Check sheet for the modelled part. Datum: model origin and axes. Units: mm. A direction names the side the tool comes from. Round coordinates to 2 decimals unless told otherwise and drop trailing zeros. Order: outer loops, then holes, each group sorted by start corner. A loop starts at its lowest first (then second) coordinate and runs counter-clockwise, first axis right, second up.
(1) Sectioned sample at B-B, the plane z = 14.5. Enter the section's corners in (x, y).
(2) Sectioned sample at C-C, the plane x = -3. Count the separate pieces of the cut face and the enclosed holes in it, and give its area (3 significant figures).
(3) Sectioned sample at A-A, the plane x = 13. Enter the section's corners in (y, z).
(4) Thickness scan on probe 1 along Z at (x, y) = (-3, 0.5) (3 decimals); probe 2 along Z at (x, y) = (-3, 1.8) (3 decimals); probe 3 along X at (y, z) = (0.45, 16.5). Record the ranges inside material, lowest first.
(5) Depth check by flat-ended pin: pin 1 (1.8 mm diameter, centred on x = -17, z = -21.285, fed in from +Y); pin 2 (3 mm diameter, centred on x = -16.77, z = -28.78, fed in from +Y). Enter the tip coordinate at first touch or a pass-through.
(6) Tool access check on faces 4 (the flat face through (-4, 1.35, 28)), 5 (the flat face through (12, 2, 26)), 6 (the flat face through (0, 0, 10)). Record the directions out of +Z, -Z, +X, -X, +Y, -Y that give a thin tool (end or side, any length) a straight path to the whole face; none if there is none.
(7) Mould release check, pull along X, two halves, no side actions. Record for faces 1 (the cylindrical face through (-16.462, 0.684, -22.128)), 2 (the flat face through (-32, 1, -1)), 3 (the flat face through (32, 1, 1)): released by +X, released by -X, zero draft, split by the parting line, or undercut.
```python
from build123d import *

# Parameters (mm, degrees)
BOSS_EXTRUDE1_DEPTH = 3
CUT_EXTRUDE2_DEPTH  = 10
SKETCH7_R           = 1
CUT_EXTRUDE3_DEPTH  = 11.5
SKETCH8_R           = 2
CUT_EXTRUDE4_DEPTH  = 1.65


with BuildPart() as part:
    # Sketch1 → Boss-Extrude1 (new body)
    with BuildSketch(Plane(origin=(0, 0, 0), x_dir=(1, 0, 0), z_dir=(0, 1, 0))):
        Polygon((-32, -43.117707706), (-20.011895516, -50), (20.011895516, -50), (32, -43.117707706), (32, 43.117707706), (20.011895516, 50), (-20.011895516, 50), (-32, 43.117707706), align=None)
    extrude(amount=BOSS_EXTRUDE1_DEPTH)

    # Sketch5 → Cut-Extrude2 (cut)
    with BuildSketch(Plane(origin=(0, 3, 0), x_dir=(1, 0, 0), z_dir=(0, 1, 0))):
        with BuildLine():
            Line((-14.620176413, -2.5), (14.620176413, -2.5))
            ThreePointArc((14.620176413, -2.5), (16.352588027, -1.782411614), (17.070176413, -0.05))
            Line((17.070176413, -0.05), (17.070176413, 0.05))
            ThreePointArc((17.070176413, 0.05), (16.352588027, 1.782411614), (14.620176413, 2.5))
            Line((14.620176413, 2.5), (-14.620176413, 2.5))
            ThreePointArc((-14.620176413, 2.5), (-16.352588027, 1.782411614), (-17.070176413, 0.05))
            Line((-17.070176413, 0.05), (-17.070176413, -0.05))
            ThreePointArc((-17.070176413, -0.05), (-16.352588027, -1.782411614), (-14.620176413, -2.5))
        make_face()
        with BuildLine():
            Line((14.45, -38.5), (14.55, -38.5))
            ThreePointArc((14.55, -38.5), (16.282411614, -37.782411614), (17, -36.05))
            Line((17, -36.05), (17, -15.95))
            ThreePointArc((17, -15.95), (16.282411614, -14.217588386), (14.55, -13.5))
            Line((14.55, -13.5), (14.45, -13.5))
            ThreePointArc((14.45, -13.5), (12.717588386, -14.217588386), (12, -15.95))
            Line((12, -15.95), (12, -36.05))
            ThreePointArc((12, -36.05), (12.717588386, -37.782411614), (14.45, -38.5))
        make_face()
        with BuildLine():
            Line((14.45, 13.5), (14.55, 13.5))
            ThreePointArc((14.55, 13.5), (16.282411614, 14.217588386), (17, 15.95))
            Line((17, 15.95), (17, 36.05))
            ThreePointArc((17, 36.05), (16.282411614, 37.782411614), (14.55, 38.5))
            Line((14.55, 38.5), (14.45, 38.5))
            ThreePointArc((14.45, 38.5), (12.717588386, 37.782411614), (12, 36.05))
            Line((12, 36.05), (12, 15.95))
            ThreePointArc((12, 15.95), (12.717588386, 14.217588386), (14.45, 13.5))
        make_face()
    extrude(amount=-CUT_EXTRUDE2_DEPTH, mode=Mode.SUBTRACT)

    # Sketch7 → Cut-Extrude3 (cut)
    with BuildSketch(Plane(origin=(0, 3, 0), x_dir=(1, 0, 0), z_dir=(0, 1, 0))):
        with Locations((-3, 28.785)):
            Circle(SKETCH7_R)
        with Locations((-3, 21.285)):
            Circle(SKETCH7_R)
        with Locations((-17, 21.285)):
            Circle(SKETCH7_R)
        with Locations((-16.76760758, 28.785)):
            Circle(SKETCH7_R)
    cut_extrude3 = extrude(amount=-CUT_EXTRUDE3_DEPTH, mode=Mode.SUBTRACT)

    # Mirror1: Cut-Extrude3 across plane
    add(cut_extrude3.mirror(Plane(origin=(0, 0, 0), x_dir=(1, 0, 0), z_dir=(0, 0, -1))), mode=Mode.SUBTRACT)

    # Sketch8 → Cut-Extrude4 (cut)
    with BuildSketch(Plane(origin=(0, 3, 0), x_dir=(1, 0, 0), z_dir=(0, 1, 0))):
        with Locations((-3, -28.785)):
            Circle(SKETCH8_R)
        with Locations((-16.76760758, -28.785)):
            Circle(SKETCH8_R)
        with Locations((-17, -21.285)):
            Circle(SKETCH8_R)
        with Locations((-3, -21.285)):
            Circle(SKETCH8_R)
        with Locations((-3, 28.785)):
            Circle(SKETCH8_R)
        with Locations((-3, 21.285)):
            Circle(SKETCH8_R)
        with Locations((-17, 21.285)):
            Circle(SKETCH8_R)
        with Locations((-16.76760758, 28.785)):
            Circle(SKETCH8_R)
    extrude(amount=-CUT_EXTRUDE4_DEPTH, mode=Mode.SUBTRACT)


solid = part.part
```
Derived:
1. outline: (-32, 0) - (12.48, 0) - (12.48, 3) - (-32, 3) - close; (16.52, 0) - (32, 0) - (32, 3) - (16.52, 3) - close
2. separate pieces: 6
2. enclosed holes: 0
2. area: 248 mm2
3. outline: (0, -50) - (3, -50) - (3, -38.02) - (0, -38.02) - close; (0, -13.98) - (3, -13.98) - (3, -2.5) - (0, -2.5) - close; (0, 2.5) - (3, 2.5) - (3, 13.98) - (0, 13.98) - close; (0, 38.02) - (3, 38.02) - (3, 50) - (0, 50) - close
4. probe 1: z = -50 to -29.785, -27.785 to -22.285, -20.285 to -2.5, 2.5 to 20.285, 22.285 to 27.785, 29.785 to 50
4. probe 2: z = -50 to -30.785, -26.785 to -23.285, -19.285 to -2.5, 2.5 to 19.285, 23.285 to 26.785, 30.785 to 50
4. probe 3: x = -32 to 12, 17 to 32
5. pin 1: passes through
5. pin 2: stops at y = 1.35
6. face 4: +Y
6. face 5: +Y, -Y
6. face 6: +Z, -Z, +X, -X, -Y
7. face 1: undercut
7. face 2: released by -X
7. face 3: released by +X
